Here's how the part is built. I have some questions about the finished solid (model axes, mm). Face numbers are marked on the shaded views. A direction names the side the tool comes from. Give positions to 0.01 mm unless a question says otherwise; leave off trailing zeros. Loops run counter-clockwise (first coordinate to the right, second up) from the corner with the lowest first, then second, coordinate; pieces in that order, holes last. Notation, with made-up numbers: M 35,67.25 L 94,67.25 A17 cw 94,81.25 Z; hole C -33,51.5 d6. An arc over 180 degrees is marked long. Answer as CSV lines item,"result". Start each with the question number.
Item 1: I want a section at D-D on x = -8.5. List the corners of the cut face in (y, z) for me.
Item 2: I want a section at A-A on z = 0. List the corners of the cut face in (x, y) for me.
Item 3: If I drill on line 1 along Y through (x, z) = (-4.25, 0); line 2 along X through (y, z) = (6.75, -6.5), over which ranges is the centre line in solid material (lowest first)? Write a range as from..to.
Item 4: I want a section at C-C on y = -4.5. List the corners of the cut face in (x, z) for me.
Item 5: Will these pins go through, and if not, where does the flat tip stop? P1, Ø5, axis at x = -10, y = 7, coming from the +Z side; P2, Ø5, axis at x = 5, y = -2.5, coming from the +Z side; P3, Ø3, axis at x = -12, z = 3.5, coming from the -Y side.
Item 6: If we mould it in two halves opening along Z, with no side actions, what happens to the marked faces 1, 2 and 3? For each: released by +Z, released by -Z, zero draft, split by the parting line, or undercut.
Item 7: For the marked faces 4 and 5, which set-ups out of +Z, -Z, +X, -X, +Y, -Y let a thin tool reach every point of the face, with its end or its side?
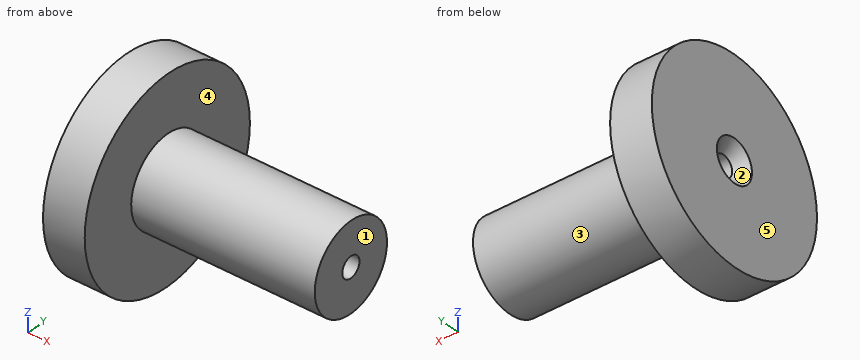
from build123d import *

# Parameters (mm, degrees)
F2_SIZE = 1.3


with BuildPart() as f1:
    # F0 (on Front) → F1 (revolve)
    with BuildSketch(Plane.XZ):
        Polygon((-17.69014, 12), (-17.69014, 1.25), (9.30986, 1.25), (9.30986, 5.25), (-12.69014, 5.25), (-12.69014, 12), align=None)
    revolve(axis=Axis((-2.74572, 0, 0), (1, 0, 0)))

    # F2
    f2_edges = [f1.edges().sort_by_distance(p)[0] for p in [
        (-17.69014, 0, -1.25),
    ]]
    chamfer(f2_edges, length=F2_SIZE)


solid = f1.part
Result:
1,outline,"C 0,0 d10.5; hole C 0,0 d2.5"
2,outline,"M -17.69,-12 L -12.69,-12 L -12.69,-5.25 L 9.31,-5.25 L 9.31,-1.25 L -16.39,-1.25 L -17.69,-2.55 Z; M -17.69,2.55 L -16.39,1.25 L 9.31,1.25 L 9.31,5.25 L -12.69,5.25 L -12.69,12 L -17.69,12 Z"
3,line 1,"-5.25..-1.25, 1.25..5.25"
3,line 2,"-17.69..-12.69"
4,outline,"M -17.69,-11.12 L -12.69,-11.12 L -12.69,-2.7 L 9.31,-2.7 L 9.31,2.7 L -12.69,2.7 L -12.69,11.12 L -17.69,11.12 Z"
5,P1,"z = 2.7"
5,P2,"z = 5.25"
5,P3,"y = -11.8"
6,face 1,"zero draft"
6,face 2,"undercut"
6,face 3,"split by the parting line"
7,face 4,"+X"
7,face 5,"+Z, -Z, -X, +Y, -Y"
